Check sheet for the modelled part. Datum: model origin and axes. Units: mm. A direction names the side the tool comes from. Round coordinates to 2 decimals unless told otherwise and drop trailing zeros. Write each loop counter-clockwise with the first axis right and the second up, starting at its lowest first coordinate (ties: lowest second). Pieces come first, ordered by that corner, then holes. Notation, with made-up numbers: (62, 66) -> (115, 66) arc R25 ccw to (115, 91) -> close; hole circle Ø2 at (-1, 45). An arc over 180 degrees is marked (long way). Put each result on its own line as item: value. Start each with the question number.
from build123d import *

# Parameters (mm, degrees)
F0_W      = 30
F0_H      = 30
F1_DEPTH  = 15
F2_R      = 2.5
F3_DEPTH  = 1
F4_R      = 2.5
F5_DEPTH  = 1
F6_R      = 2.5
F7_DEPTH  = 1
F8_R      = 2.5
F9_DEPTH  = 1
F10_R     = 2.5
F11_DEPTH = 1
F12_R     = 2.5
F13_DEPTH = 1
F14_R     = 5


with BuildPart() as f1:
    # F0 (on Front) → F1 (new body, symmetric)
    with BuildSketch(Plane.XZ):
        Rectangle(F0_W, F0_H)
    extrude(amount=F1_DEPTH, both=True)

    # F2 (on face) → F3 (cut)
    with BuildSketch(Plane.XZ.offset(15)):
        Circle(F2_R)
    extrude(amount=-F3_DEPTH, mode=Mode.SUBTRACT)

    # F4 (on face) → F5 (cut)
    with BuildSketch(Plane(origin=(0, 15, 0), x_dir=(-1, 0, 0), z_dir=(0, 1, 0))):
        with Locations((-7, 7)):
            Circle(F4_R)
        with Locations((-7, 0)):
            Circle(F4_R)
        with Locations((-7, -7)):
            Circle(F4_R)
        with Locations((7, -7)):
            Circle(F4_R)
        with Locations((7, 0)):
            Circle(F4_R)
        with Locations((7, 7)):
            Circle(F4_R)
    extrude(amount=-F5_DEPTH, mode=Mode.SUBTRACT)

    # F6 (on face) → F7 (cut)
    with BuildSketch(Plane.YZ.offset(15)):
        with Locations((-7, 7)):
            Circle(F6_R)
        Circle(F6_R)
        with Locations((7, -7)):
            Circle(F6_R)
    extrude(amount=-F7_DEPTH, mode=Mode.SUBTRACT)

    # F8 (on face) → F9 (cut)
    with BuildSketch(Plane(origin=(-15, 0, 0), x_dir=(0, -1, 0), z_dir=(-1, 0, 0))):
        with Locations((-7, 7)):
            Circle(F8_R)
        with Locations((7, 7)):
            Circle(F8_R)
        with Locations((7, -7)):
            Circle(F8_R)
        with Locations((-7, -7)):
            Circle(F8_R)
    extrude(amount=-F9_DEPTH, mode=Mode.SUBTRACT)

    # F10 (on face) → F11 (cut)
    with BuildSketch(Plane.XY.offset(15)):
        with Locations((6.801882, -6.998598)):
            Circle(F10_R)
        with Locations((-7.198118, -6.998598)):
            Circle(F10_R)
        Circle(F10_R)
        with Locations((7, 7)):
            Circle(F10_R)
        with Locations((-7, 7)):
            Circle(F10_R)
    extrude(amount=-F11_DEPTH, mode=Mode.SUBTRACT)

    # F12 (on face) → F13 (cut)
    with BuildSketch(Plane(origin=(0, 0, -15), x_dir=(1, 0, 0), z_dir=(0, 0, -1))):
        with Locations((-7, 7)):
            Circle(F12_R)
        with Locations((7, -7)):
            Circle(F12_R)
    extrude(amount=-F13_DEPTH, mode=Mode.SUBTRACT)

    # F14
    f14_edges = [f1.edges().sort_by_distance(p)[0] for p in [
        (-15, 0, 15),
        (-15, 15, 0),
        (-15, -15, 0),
        (-15, 0, -15),
        (0, -15, -15),
        (0, -15, 15),
        (15, -15, 0),
        (0, 15, -15),
        (15, 0, -15),
        (0, 15, 15),
        (15, 0, 15),
        (15, 15, 0),
    ]]
    fillet(f14_edges, radius=F14_R)


solid = f1.part
1. Section check B-B, the plane y = 0.75. Enter the section's corners in (x, z).
2. Section check A-A, the plane z = 7. Enter the section's corners in (x, y), then the cut area to 3 significant figures.
3. Section check D-D, the plane z = 0. Enter the section's corners in (x, y).
4. Access from +Z, -Z, +X, -X, +Y, -Y to the whole of each face (thin tool, end or side, straight path). Record for faces 1 (the cylindrical face through (9.31, 7.96, -14.51)), 2 (the cylindrical face through (6.26, -9.44, 14.51)), 3 (the flat face through (-14, -7, 7)), 4 (the cylindrical face through (4.615, 14.507, 0.751)).
5. Gauge pin test, flat ends, axial feed: P1, Ø2.5, axis at y = -1, z = 0, coming from the +X side; P2, Ø1.5, axis at y = -7.5, z = 7.5, coming from the -X side; P3, Ø2.5, axis at x = -8, z = -7, coming from the +Y side. Record the tip position at first contact, or that the pin passes through.
6. Material ranges on L1, parallel to Z at x = -14.6, y = 7; L2, parallel to Z at x = -7, y = 14.6; L3, parallel to Z at x = 7.5, y = -7.5, recorded low to high. Write a range as [from, to].
7. Draft check along X on faces 5 (the flat face through (-2, -15, -2)), 6 (the cylindrical face through (-14, -13, 0)), 7 (the cylindrical face through (-9.385, 14.507, 0.751)). Enter one of: released by +X, released by -X, zero draft, split by the parting line, or undercut.
Reply:
1. outline: (-15, -10) arc R5 ccw to (-10, -15) -> (10, -15) arc R5 ccw to (15, -10) -> (15, -2.38) -> (14, -2.38) -> (14, 2.38) -> (15, 2.38) -> (15, 10) arc R5 ccw to (10, 15) -> (2.38, 15) -> (2.38, 14) -> (-2.38, 14) -> (-2.38, 15) -> (-10, 15) arc R5 ccw to (-15, 10) -> close
2. outline: (-15, -10) arc R5 ccw to (-10, -15) -> (10, -15) arc R5 ccw to (15, -10) -> (15, -9.5) -> (14, -9.5) -> (14, -4.5) -> (15, -4.5) -> (15, 10) arc R5 ccw to (10, 15) -> (9.5, 15) -> (9.5, 14) -> (4.5, 14) -> (4.5, 15) -> (-4.5, 15) -> (-4.5, 14) -> (-9.5, 14) -> (-9.5, 15) -> (-10, 15) arc R5 ccw to (-15, 10) -> (-15, 9.5) -> (-14, 9.5) -> (-14, 4.5) -> (-15, 4.5) -> (-15, -4.5) -> (-14, -4.5) -> (-14, -9.5) -> (-15, -9.5) -> close
2. area: 854 mm2
3. outline: (-15, -10) arc R5 ccw to (-10, -15) -> (-2.5, -15) -> (-2.5, -14) -> (2.5, -14) -> (2.5, -15) -> (10, -15) arc R5 ccw to (15, -10) -> (15, -2.5) -> (14, -2.5) -> (14, 2.5) -> (15, 2.5) -> (15, 10) arc R5 ccw to (10, 15) -> (9.5, 15) -> (9.5, 14) -> (4.5, 14) -> (4.5, 15) -> (-4.5, 15) -> (-4.5, 14) -> (-9.5, 14) -> (-9.5, 15) -> (-10, 15) arc R5 ccw to (-15, 10) -> close
4. face 1: -Z
4. face 2: +Z
4. face 3: -X
4. face 4: +Y
5. P1: stops at x = 14
5. P2: stops at x = -14
5. P3: stops at y = 14
6. L1: z = [-11.96, -9.5], [-4.5, 4.5], [9.5, 11.96]
6. L2: z = [-11.96, -9.5], [-4.5, -2.5], [2.5, 4.5], [9.5, 11.96]
6. L3: z = [-15, 14]
7. face 5: zero draft
7. face 6: released by -X
7. face 7: undercut
